The drawing under review shows one solid part. Ordinate dimensions are in mm from its lowest x, y, z. A direction names the side the tool comes from. Give positions to 0.01 mm unless a question says otherwise; leave off trailing zeros. Write each loop counter-clockwise with the first axis right and the second up, starting at its lowest first coordinate (ties: lowest second). Pieces come first, ordered by that corner, then holes. Notation, with made-up numbers: M 31.5,15 L 85.5,15 A23 ccw 85.5,49 Z; hole C 35.25,-31 d10. An arc over 180 degrees is marked long. Write each question's results on one line, items separated by ' | '. Start each with the question number.
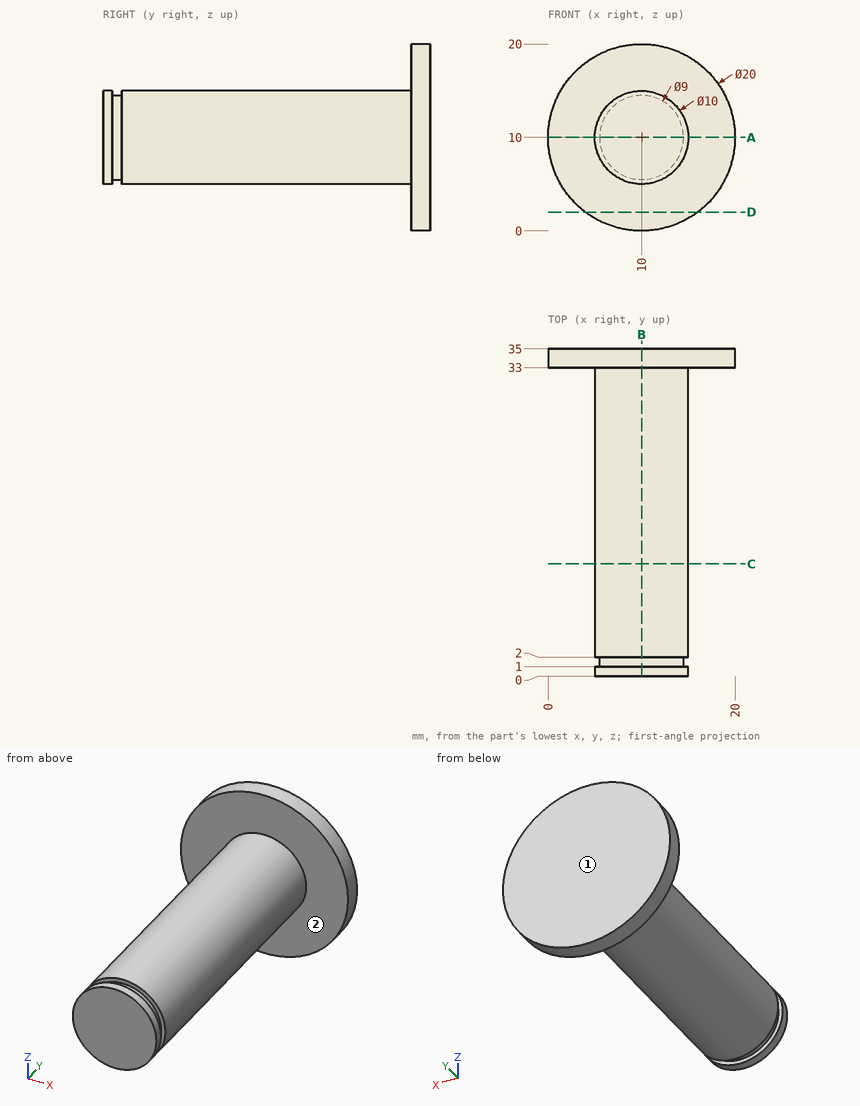
Q1. We need section D-D on z = 2. Write out the cut boundary in (x, y), and give its area (3 significant figures).
Q2. Wall thickness on line 1 along X through (y, z) = (29, 9.75); line 2 along Y through (x, z) = (16.25, 16.25); line 3 along Y through (x, z) = (7.5, 6): over which ranges is each line inside the solid? List them lowest first. Write a range as from..to.
Q3. We need section A-A on z = 10. Write out the cut boundary in (x, y).
Q4. We need section C-C on y = 12. Write out the cut boundary in (x, z).
Q5. We need section B-B on x = 10. Write out the cut boundary in (y, z).
Q6. For pin 1 Ø4 at (x, y) = (13.5, 4) entering from +Z; pin 2 Ø8 at (x, y) = (4.5, 5.5) entering from -Z; pin 3 Ø10 at (y, z) = (18.5, 11) entering from +X, all flat-tipped, find the tip position at first contact; note any pin that passes through.
Q7. For the marked faces 1 and 2, list the 3-axis set-ups (+Z, -Z, +X, -X, +Y, -Y) from which the entire face can be reached by the end or side of a thin tool; tool diameter is ignored.
Answer sheet:
1) outline: M 4,33 L 16,33 L 16,35 L 4,35 Z | area: 24.0 mm^2
2) line 1: 5.01..14.99 | line 2: 33..35 | line 3: 0..1, 2..35
3) outline: M 0,33 L 5,33 L 5,2 L 5.5,2 L 5.5,1 L 5,1 L 5,0 L 15,0 L 15,1 L 14.5,1 L 14.5,2 L 15,2 L 15,33 L 20,33 L 20,35 L 0,35 Z
4) outline: C 10,10 d10
5) outline: M 0,5 L 1,5 L 1,5.5 L 2,5.5 L 2,5 L 33,5 L 33,0 L 35,0 L 35,20 L 33,20 L 33,15 L 2,15 L 2,14.5 L 1,14.5 L 1,15 L 0,15 Z
6) pin 1: z = 14.77 | pin 2: z = 5.23 | pin 3: x = 15
7) face 1: +Z, -Z, +X, -X, +Y | face 2: -Y
